```python
from build123d import *

# Parameters (mm, degrees)
F0_R     = 39
F0_R_2   = 4.6
F1_DEPTH = 3


with BuildPart() as f1:
    # F0 (on Top) → F1 (new body)
    with BuildSketch(Plane.XY):
        with BuildLine():
            ThreePointArc((0, 11), (-7.778175, -7.778175), (11, 0))
            ThreePointArc((11, 0), (7.778175, 7.778175), (0, 11))
        make_face()
        with BuildLine():
            ThreePointArc((4.6, 31), (-3.252691, 34.252691), (0, 26.4))
            ThreePointArc((0, 26.4), (3.252691, 27.747309), (4.6, 31))
        make_face()
        Circle(F0_R)
        with Locations((-21.92031, -21.92031)):
            Circle(F0_R_2, mode=Mode.SUBTRACT)
        with Locations((-13.435029, -13.435029)):
            Circle(F0_R_2, mode=Mode.SUBTRACT)
        with Locations((0, -31)):
            Circle(F0_R_2, mode=Mode.SUBTRACT)
        with Locations((21.92031, -21.92031)):
            Circle(F0_R_2, mode=Mode.SUBTRACT)
        with Locations((0, -19)):
            Circle(F0_R_2, mode=Mode.SUBTRACT)
        with Locations((13.435029, -13.435029)):
            Circle(F0_R_2, mode=Mode.SUBTRACT)
        with Locations((-31, 0)):
            Circle(F0_R_2, mode=Mode.SUBTRACT)
        with Locations((-19, 0)):
            Circle(F0_R_2, mode=Mode.SUBTRACT)
        with Locations((-13.435029, 13.435029)):
            Circle(F0_R_2, mode=Mode.SUBTRACT)
        with Locations((-21.92031, 21.92031)):
            Circle(F0_R_2, mode=Mode.SUBTRACT)
        with BuildLine():
            ThreePointArc((0, 11), (7.778175, 7.778175), (11, 0))
            ThreePointArc((11, 0), (-7.778175, -7.778175), (0, 11))
        make_face(mode=Mode.SUBTRACT)
        with Locations((19, 0)):
            Circle(F0_R_2, mode=Mode.SUBTRACT)
        with BuildLine():
            ThreePointArc((4.6, 19), (3.252691, 15.747309), (0, 14.4))
            ThreePointArc((0, 14.4), (-4.6, 19), (0, 23.6))
            ThreePointArc((0, 23.6), (3.252691, 22.252691), (4.6, 19))
        make_face(mode=Mode.SUBTRACT)
        with Locations((13.435029, 13.435029)):
            Circle(F0_R_2, mode=Mode.SUBTRACT)
        with Locations((31, 0)):
            Circle(F0_R_2, mode=Mode.SUBTRACT)
        with BuildLine():
            ThreePointArc((4.6, 31), (3.252691, 27.747309), (0, 26.4))
            ThreePointArc((0, 26.4), (-3.252691, 34.252691), (4.6, 31))
        make_face(mode=Mode.SUBTRACT)
        with Locations((21.92031, 21.92031)):
            Circle(F0_R_2, mode=Mode.SUBTRACT)
    extrude(amount=F1_DEPTH)


solid = f1.part
```
Input: part model. Units: mm. Frame: model coordinates. Coordinates: 2 decimals unless noted, no trailing zeros. Write each loop counter-clockwise with the first axis right and the second up, starting at its lowest first coordinate (ties: lowest second). Pieces come first, ordered by that corner, then holes. Notation, with made-up numbers: (10, -30.75) -> (64, -30.75) arc R27 cw to (64, -1.75) -> close; hole circle Ø11 at (-23, -38.5). An arc over 180 degrees is marked (long way). Answer as a JSON object with one key per item and string values.
1. Section B-B on y = 2.5. Return the cut outline in (x, z), then the cut area to 3 significant figures.
Result set:
{"outline": "(-38.92, 0) -> (-34.86, 0) -> (-34.86, 3) -> (-38.92, 3) -> close; (-27.14, 0) -> (-22.86, 0) -> (-22.86, 3) -> (-27.14, 3) -> close; (-15.14, 0) -> (-10.71, 0) -> (-10.71, 3) -> (-15.14, 3) -> close; (10.71, 0) -> (15.14, 0) -> (15.14, 3) -> (10.71, 3) -> close; (22.86, 0) -> (27.14, 0) -> (27.14, 3) -> (22.86, 3) -> close; (34.86, 0) -> (38.92, 0) -> (38.92, 3) -> (34.86, 3) -> close", "area": "76.6 mm2"}
2. Material intervals for line 1 (Y direction, x = -3.5, z = 2.4); line 2 (Y direction, x = -13.5, z = 2.05); line 3 (Y direction, x = 25.5, z = 2), sorted ascending. Write a range as from..to.
Result set:
{"line 1": "y = -38.84..-33.98, -28.02..-21.98, -16.02..-10.43, 10.43..16.02, 21.98..28.02, 33.98..38.84", "line 2": "y = -36.59..-18.03, -8.84..8.84, 18.03..36.59", "line 3": "y = -29.51..-24.81, -19.03..19.03, 24.81..29.51"}
3. Section A-A on x = 29.5. Return the cut outline in (y, z), then the cut area to 3 significant figures.
Result set:
{"outline": "(-25.51, 0) -> (-4.35, 0) -> (-4.35, 3) -> (-25.51, 3) -> close; (4.35, 0) -> (25.51, 0) -> (25.51, 3) -> (4.35, 3) -> close", "area": "127 mm2"}
4. First-contact query: P1, Ø1, axis at x = 15.5, z = 1, coming from the +Y side. Flat tip, straight axial feed; report the tip coordinate or a pass-through.
Result set:
{"P1": "stops at y = 36"}
5. Mould query, pull axis X, two halves, no side actions, for faces 1 (the face through (8, -8, 0)), 2 (the face through (-23.596, 0.202, 1.479)), 3 (the face through (-5.077, 38.668, 1.479)). Classes: released by +X, released by -X, zero draft, split by the parting line, or undercut.
Result set:
{"face 1": "zero draft", "face 2": "undercut", "face 3": "split by the parting line"}
6. Section D-D on y = 33.5. Return the cut outline in (x, z), then the cut area to 3 significant figures.
Result set:
{"outline": "(-19.97, 0) -> (-3.86, 0) -> (-3.86, 3) -> (-19.97, 3) -> close; (3.86, 0) -> (19.97, 0) -> (19.97, 3) -> (3.86, 3) -> close", "area": "96.6 mm2"}
7. Section C-C on z = 2. Count the separate pieces of the cut face and the enclosed holes in it, then the cut area to 3 significant figures.
Result set:
{"separate pieces": "1", "enclosed holes": "17", "area": "3,330 mm2"}
